Input: part model. Units: mm. Frame: model coordinates. Face numbers are marked on the shaded views. Give positions to 0.01 mm unless a question says otherwise; leave off trailing zeros. Loops run counter-clockwise (first coordinate to the right, second up) from the corner with the lowest first, then second, coordinate; pieces in that order, holes last. Notation, with made-up numbers: M 86,81 L 106,81 A19 ccw 106,101 Z; hole C 87,-35.75 d1. An arc over 180 degrees is marked long. Use CSV: the item, a comma, the result in double quotes. Start each with the question number.
from build123d import *

# Parameters (mm, degrees)
SKETCH_1_W               = 12
SKETCH_1_H               = 12
EXTRUDE_1_DEPTH          = 8
FILLET_1_R               = 2.5
SKETCH_2_R               = 4.5
CUT_EXTRUDE_1_DEPTH      = 0.1
SKETCH_3_R               = 1.25
CUT_EXTRUDE_2_DEPTH      = 0.1
PATTERN_CIRCULAR_1_COUNT = 4


with BuildPart() as part:
    # Sketch 1 → Extrude 1 (new body)
    with BuildSketch(Plane.XY):
        Rectangle(SKETCH_1_W, SKETCH_1_H)
    extrude(amount=EXTRUDE_1_DEPTH)

    # Fillet 1
    fillet_1_edges = [part.edges().sort_by_distance(p)[0] for p in [
        (6, -6, 4),
        (-6, -6, 4),
        (-6, 6, 4),
        (6, 6, 4),
    ]]
    fillet(fillet_1_edges, radius=FILLET_1_R)

    # Sketch 2 → Cut-Extrude 1 (cut)
    with BuildSketch(Plane.XY.offset(8)):
        Circle(SKETCH_2_R)
    extrude(amount=-CUT_EXTRUDE_1_DEPTH, mode=Mode.SUBTRACT)

    # Sketch 3 → Cut-Extrude 2 (cut)
    with BuildSketch(Plane.XY.offset(8)):
        with Locations((-3.7, -3.7)):
            Circle(SKETCH_3_R)
    cut_extrude_2 = extrude(amount=-CUT_EXTRUDE_2_DEPTH, mode=Mode.SUBTRACT)

    # Pattern Circular 1: Cut-Extrude 2 ×4 about axis
    pattern_circular_1_axis = Axis((0, 0, 0), (0, 0, 1))
    for i in range(1, PATTERN_CIRCULAR_1_COUNT):
        add(cut_extrude_2.rotate(pattern_circular_1_axis, i * 360 / PATTERN_CIRCULAR_1_COUNT), mode=Mode.SUBTRACT)


solid = part.part
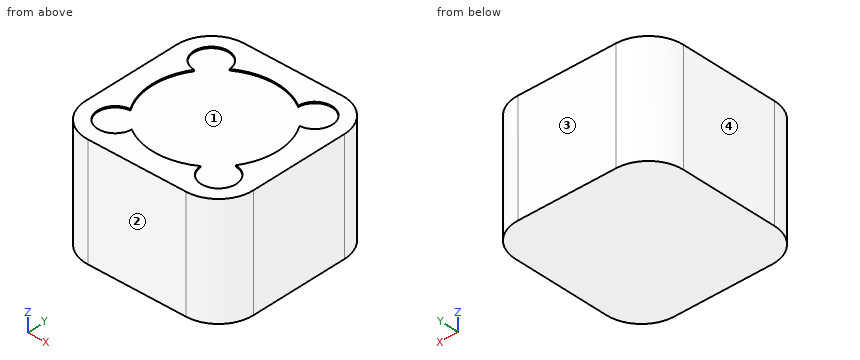
Item 1: First-contact query: pin 1 Ø2 at (x, y) = (3.7, 3.7) entering from +Z. Flat tip, straight axial feed; report the tip coordinate or a pass-through.
Item 2: Section C-C (y = -4.25). Output: boundary loops of the cut face in (x, z), then the cut area to 3 significant figures.
Item 3: Section B-B (x = -4). Output: boundary loops of the cut face in (y, z), then the cut area to 3 significant figures.
Item 4: Mould query, pull axis Y, two halves, no side actions, for the marked faces 1, 2, 3 and 4. Classes: +Y half, -Y half, draft (parallel to the pull), parting line (faces both ways), or undercut.
Item 5: Section A-A (z = 2). Output: boundary loops of the cut face in (x, y), then the cut area to 3 significant figures.
Item 6: Material intervals for line 1 (Z direction, x = 3.75, y = -3.5); line 2 (Y direction, x = 3.7, z = 7.95), sorted ascending.
Recorded:
1,pin 1,"z = 7.9"
2,outline,"M -5.88,0 L 5.88,0 L 5.88,8 L 4.82,8 L 4.82,7.9 L 2.58,7.9 L 2.58,8 L 1.48,8 L 1.48,7.9 L -1.48,7.9 L -1.48,8 L -2.58,8 L -2.58,7.9 L -4.82,7.9 L -4.82,8 L -5.88,8 Z"
2,area,"93.4 mm²"
3,outline,"M -5.95,0 L 5.95,0 L 5.95,8 L 4.91,8 L 4.91,7.9 L 2.49,7.9 L 2.49,8 L 2.06,8 L 2.06,7.9 L -2.06,7.9 L -2.06,8 L -2.49,8 L -2.49,7.9 L -4.91,7.9 L -4.91,8 L -5.95,8 Z"
3,area,"94.3 mm²"
4,face 1,"undercut"
4,face 2,"-Y half"
4,face 3,"+Y half"
4,face 4,"draft"
5,outline,"M -6,-3.5 A2.5 ccw -3.5,-6 L 3.5,-6 A2.5 ccw 6,-3.5 L 6,3.5 A2.5 ccw 3.5,6 L -3.5,6 A2.5 ccw -6,3.5 Z"
5,area,"139 mm²"
6,line 1,"0 to 7.9"
6,line 2,"-5.99 to -4.95, 4.95 to 5.99"
